Read the model definition and answer for the solid it produces. Units are mm, in the model's axes. A direction names the side the tool comes from. Give positions to 0.01 mm unless a question says otherwise; leave off trailing zeros. Order: outer loops, then holes, each group sorted by start corner. A loop starts at its lowest first (then second) coordinate and runs counter-clockwise, first axis right, second up. Notation, with made-up numbers: (38, 12.25) - (82, 12.25) arc R9 cw to (82, 19.25) - close; hole circle Ø9 at (-26.5, 50). An arc over 180 degrees is marked (long way). Use a Markdown table: item, result. Add a question column.
1. Which of the six approach directions +Z, -Z, +X, -X, +Y, -Y give full straight-line access (tool end or side, diameter ignored) to faces 1 (the flat face through (163, 4, 7)), 2 (the flat face through (0, 44, 6))?
2. Flat-ended cylindrical pins translate along their axes: P1, Ø3, axis at x = 123, z = 5, coming from the -Y side; P2, Ø4.5, axis at x = 120, z = 8.5, coming from the +Y side; P3, Ø5, axis at x = 5.5, y = 20, coming from the -Z side. Find the tip coordinate at first contact, or state that the pin passes through.
3. Consider L1, parallel to X at y = 82.5, z = 8.5; L2, parallel to Z at x = 30, y = 27; L3, parallel to X at y = 20, z = 6.25. Determine where each line is inside the solid, lowest interval first.
4. A cutting plane is placed at B-B on x = 254.5. Determine the outline of the cut face in (y, z).
5. A cutting plane is placed at A-A on z = 5. Determine the outline of the cut face in (x, y), and give its area (3 significant figures).
6. For a pull along Y with two mould halves and no side action, classify faces 3 (the conical face through (321.25, 21.6, 2.33)), 4 (the flat face through (163, 86, 7)), 5 (the flat face through (330, 44, 7)) as released by +Y, released by -Y, zero draft, split by the parting line, or undercut.
```python
from build123d import *

# Parameters (mm, degrees)
SKETCH_1_W                     = 330
SKETCH_1_H                     = 90
EXTRUDE_1_DEPTH                = 12
SKETCH_2_W                     = 9
SKETCH_2_H                     = 4
CUT_EXTRUDE_1_DEPTH            = 331
FILLET_1_R                     = 2
FILLET_2_R                     = 2
HOLE_WIZARD_M4_1_D             = 3.3
HOLE_WIZARD_M4_1_2_D           = 4.5
HOLE_WIZARD_M4_1_2_CSINK_D     = 9.4
HOLE_WIZARD_M4_1_2_CSINK_ANGLE = 90


with BuildPart() as part:
    # 草圖1 → 填料-伸長1 (new body)
    with BuildSketch(Plane.XY):
        with Locations((165, 45)):
            Rectangle(SKETCH_1_W, SKETCH_1_H)
    extrude(amount=EXTRUDE_1_DEPTH)

    # 草圖2 → 除料-伸長1 (cut, through all)
    with BuildSketch(Plane.ZY):
        with Locations((7.5, 88)):
            Rectangle(SKETCH_2_W, SKETCH_2_H)
        with Locations((7.5, 2)):
            Rectangle(SKETCH_2_W, SKETCH_2_H)
    extrude(amount=-CUT_EXTRUDE_1_DEPTH, mode=Mode.SUBTRACT)

    # 圓角1
    fillet_1_edges = [part.edges().sort_by_distance(p)[0] for p in [
        (165, 90, 0),
        (165, 0, 0),
    ]]
    fillet(fillet_1_edges, radius=FILLET_1_R)

    # 圓角2
    fillet_2_edges = [part.edges().sort_by_distance(p)[0] for p in [
        (330, 90, 2.5),
        (330, 0, 2.5),
        (330, 45, 0),
        (330, 89.414213562, 0.585786438),
        (330, 0.585786438, 0.585786438),
    ]]
    fillet(fillet_2_edges, radius=FILLET_2_R)

    # Hole Wizard M4 _1 (through all)
    with Locations(Plane(origin=(0, 86, 0), x_dir=(1, 0, 0), z_dir=(0, 1, 0))):
        with Locations((30, -8.5), (120, -8.5), (210, -8.5), (300, -8.5)):
            Hole(HOLE_WIZARD_M4_1_D / 2)

    # Hole Wizard M4 _1 2 (through all)
    with Locations(Plane(origin=(0, 0, 0), x_dir=(-1, 0, 0), z_dir=(0, 0, -1))):
        with Locations((-323, 20), (-323, 70), (-5.5, 20), (-5.5, 70)):
            CounterSinkHole(HOLE_WIZARD_M4_1_2_D / 2, HOLE_WIZARD_M4_1_2_CSINK_D / 2, counter_sink_angle=HOLE_WIZARD_M4_1_2_CSINK_ANGLE)


solid = part.part
```
Output values:
| question | item | result |
|---|---|---|
| 1 | face 1 | +Z, +X, -X, -Y |
| 1 | face 2 | +Z, -Z, -X, +Y, -Y |
| 2 | P1 | y = 4 |
| 2 | P2 | y = 86 |
| 2 | P3 | z = 2.2 |
| 3 | L1 | 0 to 28.35, 31.65 to 118.35, 121.65 to 208.35, 211.65 to 298.35, 301.65 to 330 |
| 3 | L2 | 0 to 6.85, 10.15 to 12 |
| 3 | L3 | 0 to 3.25, 7.75 to 320.75, 325.25 to 330 |
| 4 | outline | (0, 2) arc R2 ccw to (2, 0) - (88, 0) arc R2 ccw to (90, 2) - (90, 3) - (86, 3) - (86, 12) - (4, 12) - (4, 3) - (0, 3) - close |
| 5 | outline | (0, 4) - (330, 4) - (330, 86) - (0, 86) - close; hole circle Ø4.5 at (5.5, 20); hole circle Ø4.5 at (5.5, 70); hole circle Ø4.5 at (323, 20); hole circle Ø4.5 at (323, 70) |
| 5 | area | 27,000 mm² |
| 6 | face 3 | undercut |
| 6 | face 4 | released by +Y |
| 6 | face 5 | zero draft |
